The listing builds one solid part. Answer for the finished solid, in the listing's coordinates (mm). A direction names the side the tool comes from. Coordinates: 2 decimals unless noted, no trailing zeros. Loops run counter-clockwise (first coordinate to the right, second up) from the corner with the lowest first, then second, coordinate; pieces in that order, holes last. Notation, with made-up numbers: M 21,-16 L 51,-16 A8 cw 51,-3 Z; hole C 86.5,73.25 d8. An arc over 180 degrees is marked long. Answer as CSV lines item,"result". Start each with the question number.
```python
from build123d import *

# Parameters (mm, degrees)
SKETCH1_R           = 50.8
BOSS_EXTRUDE1_DEPTH = 304.8
SKETCH2_W           = 101.6
SKETCH2_H           = 203.2
BOSS_EXTRUDE2_DEPTH = 50.8
FILLET1_R           = 12.7


with BuildPart() as part:
    # Sketch1 → Boss-Extrude1 (new body)
    with BuildSketch(Plane(origin=(0, 0, 0), x_dir=(1, 0, 0), z_dir=(0, 1, 0))):
        with Locations(Location((0, 0, 0), (0, 0, 90))):
            Circle(SKETCH1_R)
    extrude(amount=BOSS_EXTRUDE1_DEPTH)

    # Sketch2 → Boss-Extrude2 (add)
    with BuildSketch(Plane(origin=(0, 0, 0), x_dir=(0, 0, -1), z_dir=(1, 0, 0))):
        with Locations((0, 152.4)):
            Rectangle(SKETCH2_W, SKETCH2_H)
    extrude(amount=BOSS_EXTRUDE2_DEPTH)

    # Fillet1
    fillet1_edges = [part.edges().sort_by_distance(p)[0] for p in [
        (0, 0, 50.8),
        (0, 304.8, 50.8),
    ]]
    fillet(fillet1_edges, radius=FILLET1_R)


solid = part.part
```
Item 1: For faces 1 (the face through (38, 50.8, 41)), 2 (the face through (38, 254, 41)), 3 (the face through (40, 50.8, -40)), 4 (the face through (40, 254, -40)), determine the directions among +Z, -Z, +X, -X, +Y, -Y from which every point of the face is accessible in a straight line to the end or side of a thin tool.
Item 2: Consider line 1 (Y direction, x = -34.5, z = 18); line 2 (X direction, y = 260, z = 2). Determine where each line is inside the solid, lowest interval first.
Item 3: Section A-A on y = 88 is taken. Determine the outline of the cut face in (x, z).
Item 4: Section B-B on y = 38 is taken. Determine the outline of the cut face in (x, z).
Item 5: Each of these flat-tipped pins is pushed along its axis until it touches: P1, Ø10, axis at y = 38.5, z = -12.5, coming from the +X side; P2, Ø4, axis at x = -39, y = 87, coming from the +Z side; P3, Ø5, axis at x = 17.5, y = 47.5, coming from the -Z side. Where does it stop, or does it pass through?
Results are:
1,face 1,"+Z, +X, -Y"
1,face 2,"+Z, +X, +Y"
1,face 3,"-Z, +X, -Y"
1,face 4,"-Z, +X, +Y"
2,line 1,"0.03 to 304.77"
2,line 2,"-50.76 to 50.76"
3,outline,"M 0,-50.8 L 50.8,-50.8 L 50.8,50.8 L 0,50.8 A50.8 ccw Z"
4,outline,"C 0,0 d101.6"
5,P1,"x = 50.24"
5,P2,"z = 34.81"
5,P3,"z = -48.53"
